Build history of the part. All positions in model axes, mm. A direction names the side the tool comes from. Give positions to 0.01 mm unless a question says otherwise; leave off trailing zeros. Loops run counter-clockwise (first coordinate to the right, second up) from the corner with the lowest first, then second, coordinate; pieces in that order, holes last. Notation, with made-up numbers: (-30, 54) -> (1, 54) arc R20 ccw to (1, 80) -> close; hole circle Ø3 at (11, 14). An arc over 180 degrees is marked (long way). Answer in a Markdown table with one row per item. Add a question column.
Autodesk Inventor part; units mm, degrees
ref_plane "YZ Plane" through (0, 0, 0) normal (1, 0, 0) x (0, 1, 0)
ref_plane "XZ Plane" through (0, 0, 0) normal (0, 1, 0) x (-1, 0, 0)
ref_plane "XY Plane" through (0, 0, 0) normal (0, 0, 1) x (1, 0, 0)
sketch "Sketch12" plane through (0, 0, 0) normal (0, 0, 1) x (1, 0, 0)
  line L0 (-12.5, 15) -> (12.5, 15)
  line L1 (12.5, 15) -> (12.5, -15)
  line L2 (12.5, -15) -> (-12.5, -15)
  line L3 (-12.5, -15) -> (-12.5, 15)
  line L4 (-12.5, 15) -> (12.5, -15) construction
  line L5 (12.5, 15) -> (-12.5, -15) construction
  point P0 (0, 0)
  dimension "d48" = 25
  dimension "d49" = 30
extrude "Extrusion12" add sketch "Sketch12" along normal blind 30
sketch "Sketch14" plane through (0, 0, 0) normal (0, 0, -1) x (-1, 0, 0)
  circle A0 centre (0, 0) radius 10.75
  dimension "d71" = 21.5
extrude "Extrusion14" cut sketch "Sketch14" against normal blind 28
sketch "Sketch15" plane through (0, 0, 30) normal (0, 0, 1) x (1, 0, 0)
  line L0 (5.75, 5.75) -> (-5.75, 5.75) construction
  line L1 (-5.75, 5.75) -> (-5.75, -5.75) construction
  line L2 (-5.75, -5.75) -> (5.75, -5.75) construction
  line L3 (5.75, -5.75) -> (5.75, 5.75) construction
  line L4 (5.75, 5.75) -> (-5.75, -5.75) construction
  line L5 (-5.75, 5.75) -> (5.75, -5.75) construction
  line L6 (5.75, 5.75) -> (2.25, 5.75)
  line L7 (2.25, 5.75) -> (2.25, -5.75)
  line L8 (2.25, -5.75) -> (5.75, -5.75)
  line L9 (5.75, -5.75) -> (5.75, 5.75)
  line L10 (-5.75, 5.75) -> (-2.25, 5.75)
  line L11 (-2.25, 5.75) -> (-2.25, -5.75)
  line L12 (-2.25, -5.75) -> (-5.75, -5.75)
  line L13 (-5.75, -5.75) -> (-5.75, 5.75)
  point P0 (0, 0)
  dimension "d74" = 11.5
  dimension "d75" = 11.5
  dimension "d76" = 3.5
  dimension "d78" = 3.5
extrude "Extrusion15" add sketch "Sketch15" along normal blind 12
sketch "Sketch16" plane through (-5.75, -5.75, 30) normal (0, -1, 0) x (1, 0, 0)
  line L0 (8, 0) -> (11.5, 0) construction
  line L1 (8, 0) -> (8, 12) construction
  line L2 (11.5, 12) -> (8, 12) construction
  line L3 (11.5, 0) -> (11.5, 12) construction
  line L4 (0, 0) -> (3.5, 0) construction
  line L5 (0, 0) -> (0, 12) construction
  line L6 (3.5, 12) -> (0, 12) construction
  line L7 (3.5, 0) -> (3.5, 12) construction
  line L8 (0, 10) -> (11.5, 10)
  line L9 (11.5, 10) -> (11.5, 7)
  line L10 (11.5, 7) -> (0, 7)
  line L11 (0, 7) -> (0, 10)
  point P0 (5.75, -30)
  dimension "d82" = 2
  dimension "d83" = 3
extrude "Extrusion16" cut sketch "Sketch16" against normal blind 5
properties part number "base"
(1) Two-plate mould, pull along Z, no slides. Class faces 1 (the flat face through (-4, 0, 42)), 2 (the flat face through (-4, -5.75, 41)), 3 (the flat face through (4, -0.75, 39)), 4 (the flat face through (-4, -3, 37)): released by +Z, released by -Z, zero draft, split by the parting line, or undercut.
(2) 3-axis set-ups, long thin cutter, end or side, ignore diameter. For faces 5 (the flat face through (2.25, 0, 36)), 6 (the flat face through (-5.75, 0, 36)), 7 (the flat face through (-4, 5.75, 36)), 8 (the flat face through (5.75, 0, 36)), 9 (the flat face through (4, -3, 40)): which of +Z, -Z, +X, -X, +Y, -Y reach the whole face in a straight line?
(3) Saw through at D-D, the plane x = 0. List the corners of the cut face in (y, z), then the cut area to 3 significant figures.
(4) Saw through at B-B, the plane y = 0. List the corners of the cut face in (x, z).
(5) Flat gauge pins, fed straight in: pin 1 Ø2 at (x, z) = (3, 40.5) entering from -Y; pin 2 Ø0.9 at (x, z) = (4, 38) entering from -Y; pin 3 Ø3 at (x, z) = (4.5, 34.5) entering from +Y. Where does each tip first touch, or does it go through?
(6) Saw through at A-A, the plane z = 33. List the corners of the cut face in (x, y), then the cut area to 3 significant figures.
(7) Wall check: line 1 along Y through (x, z) = (0, 10.5); line 2 along X through (y, z) = (4.75, 32.5); line 3 along Z through (x, y) = (-1.5, -10.25). Give the ranges that are in metal, low to high. Write a range as from..to.
(8) Saw through at C-C, the plane z = 6.5. List the corners of the cut face in (x, y), then the cut area to 3 significant figures.
Worked answers:
| question | item | result |
|---|---|---|
| 1 | face 1 | released by +Z |
| 1 | face 2 | zero draft |
| 1 | face 3 | undercut |
| 1 | face 4 | undercut |
| 2 | face 5 | +Z, +Y, -Y |
| 2 | face 6 | +Z, -X, +Y, -Y |
| 2 | face 7 | +Z, +X, -X, +Y |
| 2 | face 8 | +Z, +X, +Y, -Y |
| 2 | face 9 | +X, -X, -Y |
| 3 | outline | (-15, 0) -> (-10.75, 0) -> (-10.75, 28) -> (10.75, 28) -> (10.75, 0) -> (15, 0) -> (15, 30) -> (-15, 30) -> close |
| 3 | area | 298 mm^2 |
| 4 | outline | (-12.5, 0) -> (-10.75, 0) -> (-10.75, 28) -> (10.75, 28) -> (10.75, 0) -> (12.5, 0) -> (12.5, 30) -> (5.75, 30) -> (5.75, 42) -> (2.25, 42) -> (2.25, 30) -> (-2.25, 30) -> (-2.25, 42) -> (-5.75, 42) -> (-5.75, 30) -> (-12.5, 30) -> close |
| 5 | pin 1 | y = -5.75 |
| 5 | pin 2 | y = -0.75 |
| 5 | pin 3 | y = 5.75 |
| 6 | outline | (-5.75, -5.75) -> (-2.25, -5.75) -> (-2.25, 5.75) -> (-5.75, 5.75) -> close; (2.25, -5.75) -> (5.75, -5.75) -> (5.75, 5.75) -> (2.25, 5.75) -> close |
| 6 | area | 80.5 mm^2 |
| 7 | line 1 | -15..-10.75, 10.75..15 |
| 7 | line 2 | -5.75..-2.25, 2.25..5.75 |
| 7 | line 3 | 28..30 |
| 8 | outline | (-12.5, -15) -> (12.5, -15) -> (12.5, 15) -> (-12.5, 15) -> close; hole circle Ø21.5 at (0, 0) |
| 8 | area | 387 mm^2 |
